Check sheet for the modelled part. Datum: model origin and axes. Units: mm. A direction names the side the tool comes from. Coordinates: 2 decimals unless noted, no trailing zeros. Loops run counter-clockwise (first coordinate to the right, second up) from the corner with the lowest first, then second, coordinate; pieces in that order, holes last. Notation, with made-up numbers: M 48.5,68 L 56.5,68 A9 cw 56.5,81 Z; hole C 18,42 d4. An arc over 180 degrees is marked long. Answer as CSV lines item,"result". Start each with the question number.
from build123d import *

# Parameters (mm, degrees)
EXTRUDE_1_DEPTH      = 26
SKETCH_3_W           = 40
SKETCH_3_H           = 36
CUT_EXTRUDE_4_DEPTH  = 20
SKETCH_4_W           = 20
SKETCH_4_H           = 20
CUT_EXTRUDE_5_DEPTH  = 25
CUT_EXTRUDE_3_DEPTH  = 8
CUT_EXTRUDE_6_DEPTH  = 8
CUT_EXTRUDE_7_DEPTH  = 16
CUT_EXTRUDE_8_DEPTH  = 16
CUT_EXTRUDE_9_DEPTH  = 6
EXTRUDE_2_DEPTH      = 12
CUT_EXTRUDE_10_DEPTH = 8


with BuildPart() as part:
    # 草图1 → 凸台-拉伸1 (new body)
    with BuildSketch(Plane.XY):
        Polygon((-34, -24), (34, -24), (44, 23), (44, 46), (-44, 46), (-44, 23), align=None)
    extrude(amount=EXTRUDE_1_DEPTH)

    # 草图3 → 切除-拉伸4 (cut)
    with BuildSketch(Plane(origin=(0, 0, 0), x_dir=(-1, 0, 0), z_dir=(0, 0, -1))):
        with Locations((0, -6)):
            Rectangle(SKETCH_3_W, SKETCH_3_H)
    extrude(amount=-CUT_EXTRUDE_4_DEPTH, mode=Mode.SUBTRACT)

    # 草图4 → 切除-拉伸5 (cut)
    with BuildSketch(Plane(origin=(0, 46, 0), x_dir=(1, 0, 0), z_dir=(0, 1, 0))):
        with Locations((33, -16)):
            Rectangle(SKETCH_4_W, SKETCH_4_H)
        with Locations((11, -16)):
            Rectangle(SKETCH_4_W, SKETCH_4_H)
        with Locations((-11, -16)):
            Rectangle(SKETCH_4_W, SKETCH_4_H)
        with Locations((-32, -16)):
            Rectangle(SKETCH_4_W, SKETCH_4_H)
    extrude(amount=-CUT_EXTRUDE_5_DEPTH, mode=Mode.SUBTRACT)

    # Sketch 3D_5 → 切除-拉伸3 (cut, symmetric)
    with BuildSketch(Plane(origin=(-26.633413551, -5.666683734, 23.004025099), x_dir=(-0.691625335103945, -0.14715432661786076, 0.7071067811865475), z_dir=(-0.2081076444648591, 0.9781059289848354, 0))):
        with BuildLine():
            Line((0, 0), (5.656854249, 5.656854249))
            Line((5.656854249, 5.656854249), (11.313708499, 0))
            ThreePointArc((11.313708499, 0), (5.656854249, -13.656854249), (0, 0))
        make_face()
    extrude(amount=CUT_EXTRUDE_3_DEPTH, both=True, mode=Mode.SUBTRACT)

    # Sketch 3D_6 → 切除-拉伸6 (cut, symmetric)
    with BuildSketch(Plane(origin=(34.478414998, -7.335832978, 14.99907516), x_dir=(0.5895982688198705, -0.12544644017993214, 0.7978954016979886), z_dir=(-0.20810764446495697, -0.9781059289848145, -6.6559639472978385e-12))):
        with BuildLine():
            Line((0, 0), (6.376045072, -8.439700449))
            Line((6.376045072, -8.439700449), (17.547318622, 0))
            Line((17.547318622, 0), (11.17127355, 8.439700449))
            Line((11.17127355, 8.439700449), (6.348906145, 14.822863662))
            Line((6.348906145, 14.822863662), (1.560795809, 11.205530619))
            ThreePointArc((1.560795809, 11.205530619), (-1.540343474, 5.926016705), (0, 0))
        make_face()
    extrude(amount=CUT_EXTRUDE_6_DEPTH, both=True, mode=Mode.SUBTRACT)

    # 草图7 → 切除-拉伸7 (cut)
    with BuildSketch(Plane(origin=(-1.664861156, 7.824847432, 0), x_dir=(0.9781059289848355, 0.2081076444648587, 0), z_dir=(0.2081076444648587, -0.9781059289848355, 0))):
        with BuildLine():
            Line((-24.556702047, 20), (-31.200844281, 16.10051891))
            ThreePointArc((-31.200844281, 16.10051891), (-33.152072653, 15.280030806), (-35.250185053, 15))
            Line((-35.250185053, 15), (-43.250185053, 15))
            Line((-43.250185053, 15), (-43.250185053, 23))
            ThreePointArc((-43.250185053, 23), (-40.3181561, 29.189965223), (-33.671267687, 30.842641134))
            Line((-33.671267687, 30.842641134), (-10.087245225, 28.492198282))
            Line((-10.087245225, 28.492198282), (-24.556702047, 20))
        make_face()
    extrude(amount=CUT_EXTRUDE_7_DEPTH, mode=Mode.SUBTRACT)

    # 草图11 → 切除-拉伸8 (cut)
    with BuildSketch(Plane(origin=(-1.664861156, -7.824847432, 0), x_dir=(0.9781059289845859, -0.2081076444660318, -1.1269708570671002e-12), z_dir=(0.20810764446603178, 0.9781059289845858, 5.296763028184159e-12))):
        with BuildLine():
            Line((31.200844283, -16.100518909), (14.333584528, -26))
            Line((14.333584528, -26), (32.666556858, -30.571318601))
            ThreePointArc((32.666556858, -30.571318601), (42.196349228, -26.968728166), (40.460809076, -16.92962956))
            Line((40.460809076, -16.92962956), (38.250185053, -14.99907516))
            Line((38.250185053, -14.99907516), (35.250185053, -15))
            ThreePointArc((35.250185053, -15), (33.152072655, -15.280030806), (31.200844283, -16.100518909))
        make_face()
    extrude(amount=CUT_EXTRUDE_8_DEPTH, mode=Mode.SUBTRACT)

    # 草图12 → 切除-拉伸9 (cut)
    with BuildSketch(Plane(origin=(0, 0, 0), x_dir=(-1, 0, 0), z_dir=(0, 0, -1))):
        with BuildLine():
            Line((34, -16), (36.935033059, -16))
            Line((36.935033059, -16), (34, -24))
            Line((34, -24), (26, -24))
            Line((26, -24), (26, -20))
            ThreePointArc((26, -20), (27.171572875, -17.171572875), (30, -16))
            Line((30, -16), (34, -16))
        make_face()
    extrude(amount=-CUT_EXTRUDE_9_DEPTH, mode=Mode.SUBTRACT)

    # 草图13 → 凸台-拉伸2 (add)
    with BuildSketch(Plane(origin=(0, 0, 0), x_dir=(-1, 0, 0), z_dir=(0, 0, -1))):
        with BuildLine():
            Line((-34, -8), (-42, -8))
            ThreePointArc((-42, -8), (-46, -12), (-42, -16))
            Line((-42, -16), (-34, -16))
            Line((-34, -16), (-34, -8))
        make_face()
    extrude(amount=-EXTRUDE_2_DEPTH)

    # 草图14 → 切除-拉伸10 (cut)
    with BuildSketch(Plane(origin=(0, 0, 0), x_dir=(-1, 0, 0), z_dir=(0, 0, -1))):
        Polygon((-37.404255319, -8), (-35.70212766, -16), (-61.438279543, -16), (-61.438279543, -8), align=None)
    extrude(amount=-CUT_EXTRUDE_10_DEPTH, mode=Mode.SUBTRACT)


solid = part.part
Item 1: Go/stop test with flat-tipped pins: pin 1 (12 mm diameter, centred on x = -1, y = -6, fed in from -Z); pin 2 (4 mm diameter, centred on x = 41.5, y = -12.5, fed in from -Z); pin 3 (10 mm diameter, centred on y = 0, z = 6.5, fed in from +X); pin 4 (3 mm diameter, centred on x = -1.5, y = 24.5, fed in from +Z). Record where each tip stops, or that it passes through.
Item 2: Release check for a two-part mould opening along X. For faces 1 (the face through (-21, 34, 16)), 2 (the face through (46, -12, 10)), 3 (the face through (33, 34, 6)), 4 (the face through (40, -8, 10)) record: released by +X, released by -X, zero draft, split by the parting line, or undercut.
Item 3: Set-up check for faces 5 (the face through (20, -6, 10)), 6 (the face through (-33, -16, 3)), 7 (the face through (11, 34, 6)), 8 (the face through (-1, 19, 0)): record each of +Z, -Z, +X, -X, +Y, -Y from which the full face is reachable in a straight line by a thin tool's end or side.
Item 4: Material ranges on line 1 (X direction, y = 27, z = 10.25); line 2 (Z direction, x = -28, y = 27.5); line 3 (Z direction, x = 1, y = 8), recorded low to high. Write a range as from..to.
Item 5: Sectioned sample at C-C, the plane x = -4. Record the boundary of the cut face in (y, z), and give its area (3 significant figures).
Item 6: Sectioned sample at A-A, the plane y = 39.5. Record the boundary of the cut face in (x, z).
Reply:
1,pin 1,"z = 20"
1,pin 2,"z = 8"
1,pin 3,"x = 40.17"
1,pin 4,"z = 26"
2,face 1,"undercut"
2,face 2,"released by +X"
2,face 3,"undercut"
2,face 4,"zero draft"
3,face 5,"-Z, -Y"
3,face 6,"-Z, -X, -Y"
3,face 7,"+Z, +Y"
3,face 8,"-Z, +X, -X, +Y, -Y"
4,line 1,"-44..-42, -22..-21, -1..1, 21..23, 43..44"
4,line 2,"0..6"
4,line 3,"20..26"
5,outline,"M -24,20 L 12,20 L 12,0 L 46,0 L 46,6 L 21,6 L 21,26 L -24,26 Z"
5,area,"600 mm²"
6,outline,"M -44,0 L 44,0 L 44,26 L 43,26 L 43,6 L 23,6 L 23,26 L 21,26 L 21,6 L 1,6 L 1,26 L -1,26 L -1,6 L -21,6 L -21,26 L -22,26 L -22,6 L -42,6 L -42,26 L -44,26 Z"
